Input: part model. Units: mm. Frame: model coordinates. Coordinates: 2 decimals unless noted, no trailing zeros. Loops run counter-clockwise (first coordinate to the right, second up) from the corner with the lowest first, then second, coordinate; pieces in that order, holes last.
(1) Section B-B, the plane z = -0.35. Return loops of the section in (x, y) (1 decimal), then the cut area to 3 significant figures.
(2) Section A-A, the plane y = 6.75. Return loops of the section in (x, z).
(3) Line query: L1, parallel to Y at x = 76.2, z = -0.9 (3 decimals); L2, parallel to X at y = 8, z = -0.85; L3, parallel to X at y = 6.75, z = -1.2. Output: solid intervals per line, ascending.
(4) Section C-C, the plane y = 3. Return loops of the section in (x, z).
```python
from build123d import *

# Parameters (mm, degrees)
SKETCH1_R          = 3.2639
BASE_FLANGE1_DEPTH = 1.51892


# Sheet-metal steps are written as plain solids
with BuildPart() as part:
    # Sketch1 → Base-Flange1 (new body)
    with BuildSketch(Plane.XY):
        with BuildLine():
            Line((0, 0), (76.2, 0))
            ThreePointArc((76.2, 0), (84.1375, 7.9375), (76.2, 15.875))
            Line((76.2, 15.875), (0, 15.875))
            Line((0, 15.875), (0, 0))
        make_face()
        with Locations((76.2, 7.9375)):
            Circle(SKETCH1_R, mode=Mode.SUBTRACT)
    extrude(amount=-BASE_FLANGE1_DEPTH)


solid = part.part
```
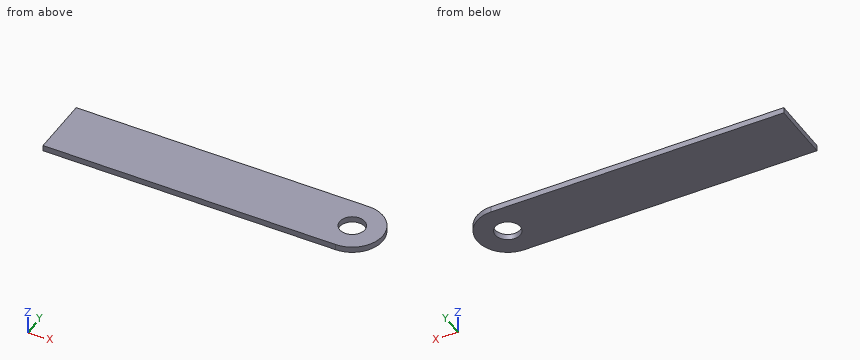
Report:
1. outline: (0, 0) - (76.2, 0) arc R7.9 ccw to (76.2, 15.9) - (0, 15.9) - close; hole circle Ø6.5 at (76.2, 7.9)
1. area: 1,280 mm2
2. outline: (0, -1.52) - (73.16, -1.52) - (73.16, 0) - (0, 0) - close; (79.24, -1.52) - (84.05, -1.52) - (84.05, 0) - (79.24, 0) - close
3. L1: y = 0 to 4.674, 11.201 to 15.875
3. L2: x = 0 to 72.94, 79.46 to 84.14
3. L3: x = 0 to 73.16, 79.24 to 84.05
4. outline: (0, -1.52) - (82.41, -1.52) - (82.41, 0) - (0, 0) - close
